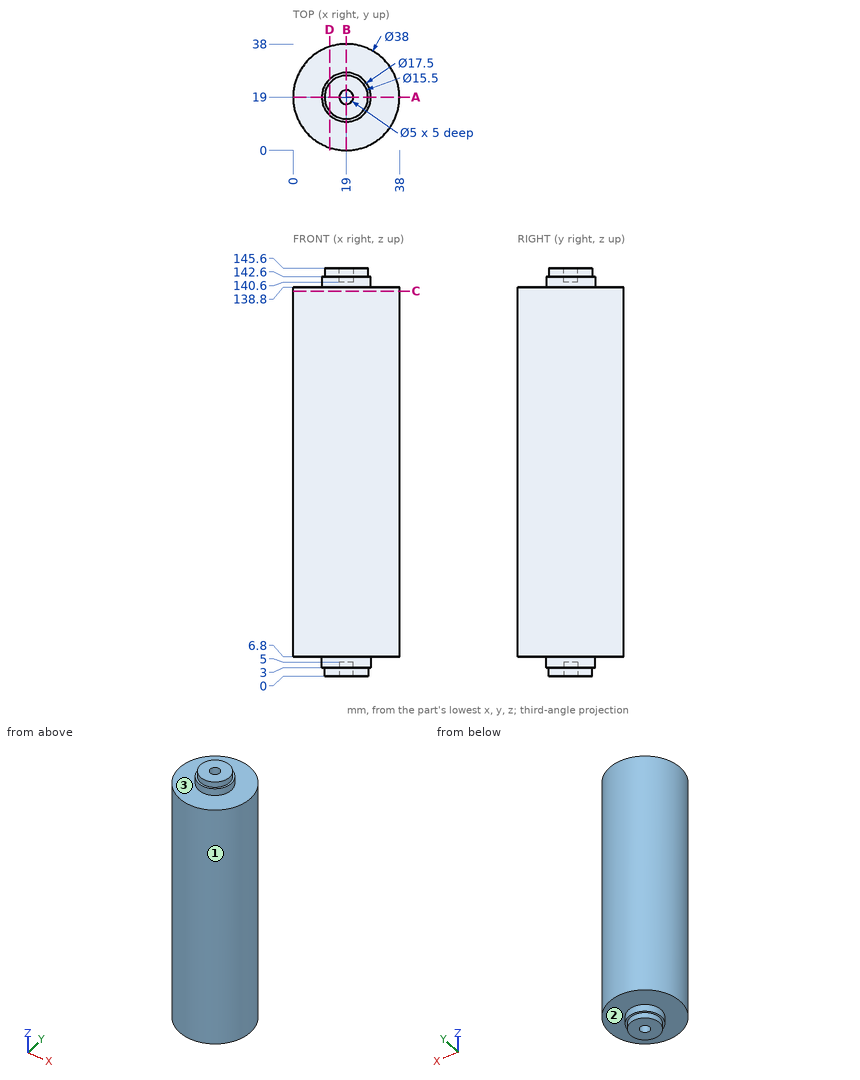
Input: dimensioned drawing with shaded views. Units: mm. Origin: part minimum x, y, z. A direction names the side the tool comes from. Give positions to 0.01 mm unless a question says otherwise; leave off trailing zeros. Loops run counter-clockwise (first coordinate to the right, second up) from the corner with the lowest first, then second, coordinate; pieces in that order, holes last. Notation, with made-up numbers: (78, 84) -> (114, 84) arc R24 ccw to (114, 115) -> close; hole circle Ø8 at (79, 64.25). An arc over 180 degrees is marked (long way). Use a Markdown table: item, result. Add a question column.
1) Section query C-C, the plane z = 137.5. Return the cut outline in (x, y).
2) Section query A-A, the plane y = 19. Return the cut outline in (x, z).
3) Line query: line 1 along Y through (x, z) = (19, 144.3); line 2 along Z through (x, y) = (15.5, 32); line 3 along X through (y, z) = (18, 134). Output: solid intervals per line, ascending. Write a range as [from, to].
4) Reachability of the marked faces 1, 2 and 3 from +Z, -Z, +X, -X, +Y, -Y: full face, straight path, thin tool, end or side. Return the list, or none.
5) First-contact query: pin 1 (6 mm diameter, centred on x = 34, z = 93.5, fed in from -Y); pin 2 (3 mm diameter, centred on x = 15, z = 82.5, fed in from -Y); pin 3 (2 mm diameter, centred on y = 33, z = 38, fed in from +X). Flat tips, straight axial feed; report the tip coordinate or a pass-through.
6) Section query D-D, the plane x = 13. Return the cut outline in (y, z), then the cut area to 4 significant figures.
Numbers:
| question | item | result |
|---|---|---|
| 1 | outline | circle Ø38 at (19, 19) |
| 2 | outline | (0, 6.8) -> (10.25, 6.8) -> (10.25, 3) -> (11.25, 3) -> (11.25, 0) -> (16.5, 0) -> (16.5, 5) -> (21.5, 5) -> (21.5, 0) -> (26.75, 0) -> (26.75, 3) -> (27.75, 3) -> (27.75, 6.8) -> (38, 6.8) -> (38, 138.8) -> (27.75, 138.8) -> (27.75, 142.6) -> (26.75, 142.6) -> (26.75, 145.6) -> (21.5, 145.6) -> (21.5, 140.6) -> (16.5, 140.6) -> (16.5, 145.6) -> (11.25, 145.6) -> (11.25, 142.6) -> (10.25, 142.6) -> (10.25, 138.8) -> (0, 138.8) -> close |
| 3 | line 1 | y = [11.25, 16.5], [21.5, 26.75] |
| 3 | line 2 | z = [6.8, 138.8] |
| 3 | line 3 | x = [0.03, 37.97] |
| 4 | face 1 | +Z, -Z |
| 4 | face 2 | -Z |
| 4 | face 3 | +Z |
| 5 | pin 1 | stops at y = 4.27 |
| 5 | pin 2 | stops at y = 0.17 |
| 5 | pin 3 | stops at x = 32.86 |
| 6 | outline | (0.97, 6.8) -> (12.63, 6.8) -> (12.63, 3) -> (14.09, 3) -> (14.09, 0) -> (23.91, 0) -> (23.91, 3) -> (25.37, 3) -> (25.37, 6.8) -> (37.03, 6.8) -> (37.03, 138.8) -> (25.37, 138.8) -> (25.37, 142.6) -> (23.91, 142.6) -> (23.91, 145.6) -> (14.09, 145.6) -> (14.09, 142.6) -> (12.63, 142.6) -> (12.63, 138.8) -> (0.97, 138.8) -> close |
| 6 | area | 4,915 mm2 |
